Source: CAD feature listing. Evaluate the final solid. Frame: model axes, mm. A direction names the side the tool comes from. Coordinates: 2 decimals unless noted, no trailing zeros. Put each result on its own line as item: value.
from build123d import *

# Parameters (mm, degrees)
SKETCH2_R          = 3.937
CUT_EXTRUDE1_DEPTH = 89.486469768
CUT_EXTRUDE2_DEPTH = 89.486469768
SKETCH5_R          = 38.857978685
SKETCH5_R_2        = 10.795
CUT_EXTRUDE3_DEPTH = 1.27
SKETCH6_R          = 9.598574497
SKETCH6_R_2        = 5.136074626
CUT_EXTRUDE4_DEPTH = 0.508
FILLET3_R          = 2.54


with BuildPart() as part:
    # Sketch1 → Revolve1 (revolve)
    with BuildSketch(Plane(origin=(0, 0, 0), x_dir=(1, 0, 0), z_dir=(0, 1, 0))):
        with BuildLine():
            Line((0, 0), (-24.13, 0))
            Line((-24.13, 0), (-24.13, 48.133))
            ThreePointArc((-24.13, 48.133), (-12.065, 60.198), (0, 48.133))
            Line((0, 48.133), (0, 0))
        make_face()
    revolve(axis=Axis((0, 0, 0), (-1, 0, 0)))

    # Sketch2 → Cut-Extrude1 (cut, through all)
    with BuildSketch(Plane(origin=(0, 0, 0), x_dir=(0, 0, -1), z_dir=(1, 0, 0))):
        Circle(SKETCH2_R)
    extrude(amount=-CUT_EXTRUDE1_DEPTH, mode=Mode.SUBTRACT)

    # Sketch3 → Cut-Extrude2 (cut, through all)
    with BuildSketch(Plane(origin=(0, 0, 0), x_dir=(0, 0, -1), z_dir=(1, 0, 0))):
        with BuildLine():
            ThreePointArc((-7.868701987, 30.719014265), (-7.414350559, 33.395529437), (-5.121198299, 34.848671341))
            ThreePointArc((-5.121198299, 34.848671341), (0, 35.222955104), (5.121198299, 34.848671341))
            ThreePointArc((5.121198299, 34.848671341), (7.414350559, 33.395529437), (7.868701987, 30.719014265))
            Line((7.868701987, 30.719014265), (5.226080148, 20.402352367))
            ThreePointArc((5.226080148, 20.402352367), (3.322663277, 17.290224183), (0, 15.784154342))
            ThreePointArc((0, 15.784154342), (-3.322663277, 17.290224183), (-5.226080148, 20.402352367))
            Line((-5.226080148, 20.402352367), (-7.868701987, 30.719014265))
        make_face()
        with BuildLine():
            Line((-16.098624321, 29.076332472), (-9.794359632, 15.986465761))
            ThreePointArc((-9.794359632, 15.986465761), (-7.273828196, 15.104584389), (-6.391946824, 17.625115825))
            Line((-6.391946824, 17.625115825), (-12.696211514, 30.714982536))
            ThreePointArc((-12.696211514, 30.714982536), (-15.216742949, 31.596863908), (-16.098624321, 29.076332472))
        make_face()
        with BuildLine():
            ThreePointArc((-12.340172279, 9.840477432), (-15.589311763, 8.181733863), (-19.209232563, 8.633962814))
            Line((-19.209232563, 8.633962814), (-28.922771395, 13.000211347))
            ThreePointArc((-28.922771395, 13.000211347), (-30.732071739, 15.024217511), (-30.438426779, 17.7230953))
            ThreePointArc((-30.438426779, 17.7230953), (-27.538038696, 21.960371467), (-24.052396954, 25.730923416))
            ThreePointArc((-24.052396954, 25.730923416), (-21.486527816, 26.61776289), (-19.11066051, 25.304209225))
            Line((-19.11066051, 25.304209225), (-12.692417211, 16.805790793))
            ThreePointArc((-12.692417211, 16.805790793), (-11.446018427, 13.377259374), (-12.340172279, 9.840477432))
        make_face()
        with BuildLine():
            Line((-32.7697437, 5.541603622), (-18.605029061, 2.309077827))
            ThreePointArc((-18.605029061, 2.309077827), (-16.344020796, 3.729864614), (-17.764807583, 5.99087288))
            Line((-17.764807583, 5.99087288), (-31.929522221, 9.223398675))
            ThreePointArc((-31.929522221, 9.223398675), (-34.190530487, 7.802611888), (-32.7697437, 5.541603622))
        make_face()
        with BuildLine():
            ThreePointArc((-15.387190118, -3.513279694), (-16.116137508, -7.087768933), (-18.726688041, -9.635976839))
            Line((-18.726688041, -9.635976839), (-28.196651006, -14.508015872))
            ThreePointArc((-28.196651006, -14.508015872), (-30.907163058, -14.660636639), (-32.834146044, -12.748332988))
            ThreePointArc((-32.834146044, -12.748332988), (-34.33861956, -7.838819794), (-35.113293701, -2.762734656))
            ThreePointArc((-35.113293701, -2.762734656), (-34.20685948, -0.203722017), (-31.698552836, 0.834818527))
            Line((-31.698552836, 0.834818527), (-21.052512511, 0.554125976))
            ThreePointArc((-21.052512511, 0.554125976), (-17.594861779, -0.60905459), (-15.387190118, -3.513279694))
        make_face()
        with BuildLine():
            Line((-24.763824671, -22.166065784), (-13.404979114, -13.107092807))
            ThreePointArc((-13.404979114, -13.107092807), (-13.106079358, -10.45351929), (-15.759652875, -10.154619535))
            Line((-15.759652875, -10.154619535), (-27.118498432, -19.213592512))
            ThreePointArc((-27.118498432, -19.213592512), (-27.417398188, -21.867166029), (-24.763824671, -22.166065784))
        make_face()
        with BuildLine():
            ThreePointArc((-6.846586936, -14.221465552), (-4.506429979, -17.020037158), (-4.141812449, -20.649829394))
            Line((-4.141812449, -20.649829394), (-6.237124282, -31.091411229))
            ThreePointArc((-6.237124282, -31.091411229), (-7.807777183, -33.305732377), (-10.504330622, -33.620006517))
            ThreePointArc((-10.504330622, -33.620006517), (-15.280766495, -31.735219868), (-19.73241109, -29.175997183))
            ThreePointArc((-19.73241109, -29.175997183), (-21.167975243, -26.87180009), (-20.416035323, -24.263207549))
            Line((-20.416035323, -24.263207549), (-13.558883477, -16.114807003))
            ThreePointArc((-13.558883477, -16.114807003), (-10.493662321, -14.136738026), (-6.846586936, -14.221465552))
        make_face()
        with BuildLine():
            Line((1.890512446, -33.182235549), (1.890046539, -18.653355221))
            ThreePointArc((1.890046539, -18.653355221), (0.001760172, -16.765189956), (-1.886405093, -18.653476323))
            Line((-1.886405093, -18.653476323), (-1.885939187, -33.182356651))
            ThreePointArc((-1.885939187, -33.182356651), (0.00234718, -35.070521916), (1.890512446, -33.182235549))
        make_face()
        with BuildLine():
            ThreePointArc((6.850388874, -14.220597785), (10.497464259, -14.135870258), (13.562685415, -16.113939236))
            Line((13.562685415, -16.113939236), (20.419837261, -24.262339782))
            ThreePointArc((20.419837261, -24.262339782), (21.171777181, -26.870932322), (19.736213028, -29.175129416))
            ThreePointArc((19.736213028, -29.175129416), (15.284568432, -31.734352101), (10.50813256, -33.619138749))
            ThreePointArc((10.50813256, -33.619138749), (7.811579121, -33.30486461), (6.240926219, -31.090543462))
            Line((6.240926219, -31.090543462), (4.145614387, -20.648961626))
            ThreePointArc((4.145614387, -20.648961626), (4.510231917, -17.019169391), (6.850388874, -14.220597785))
        make_face()
        with BuildLine():
            Line((27.122008151, -19.211505151), (15.762581618, -10.153260695))
            ThreePointArc((15.762581618, -10.153260695), (13.109027277, -10.452330638), (13.408097219, -13.105884979))
            Line((13.408097219, -13.105884979), (24.767523753, -22.164129435))
            ThreePointArc((24.767523753, -22.164129435), (27.421078094, -21.865059493), (27.122008151, -19.211505151))
        make_face()
        with BuildLine():
            ThreePointArc((15.389635159, -3.511329838), (17.597306821, -0.607104734), (21.054957553, 0.556075831))
            Line((21.054957553, 0.556075831), (31.700997878, 0.836768383))
            ThreePointArc((31.700997878, 0.836768383), (34.209304522, -0.201772161), (35.115738743, -2.7607848))
            ThreePointArc((35.115738743, -2.7607848), (34.341064602, -7.836869939), (32.836591086, -12.746383132))
            ThreePointArc((32.836591086, -12.746383132), (30.9096081, -14.658686784), (28.199096048, -14.506066016))
            Line((28.199096048, -14.506066016), (18.729133083, -9.634026983))
            ThreePointArc((18.729133083, -9.634026983), (16.11858255, -7.085819077), (15.389635159, -3.511329838))
        make_face()
        with BuildLine():
            Line((31.930831552, 9.225880469), (17.766324261, 5.992446224))
            ThreePointArc((17.766324261, 5.992446224), (16.345682487, 3.73134684), (18.606781871, 2.310705066))
            Line((18.606781871, 2.310705066), (32.771289161, 5.544139311))
            ThreePointArc((32.771289161, 5.544139311), (34.191930935, 7.805238695), (31.930831552, 9.225880469))
        make_face()
        with BuildLine():
            ThreePointArc((12.340925299, 9.842041095), (11.446771448, 13.378823037), (12.693170232, 16.807354456))
            Line((12.693170232, 16.807354456), (19.111413531, 25.305772888))
            ThreePointArc((19.111413531, 25.305772888), (21.487280836, 26.619326553), (24.053149974, 25.732487079))
            ThreePointArc((24.053149974, 25.732487079), (27.538791716, 21.96193513), (30.4391798, 17.724658963))
            ThreePointArc((30.4391798, 17.724658963), (30.732824759, 15.025781174), (28.923524416, 13.00177501))
            Line((28.923524416, 13.00177501), (19.209985583, 8.635526477))
            ThreePointArc((19.209985583, 8.635526477), (15.590064784, 8.183297526), (12.340925299, 9.842041095))
        make_face()
        with BuildLine():
            Line((12.695840543, 30.715989922), (6.392415389, 17.625718912))
            ThreePointArc((6.392415389, 17.625718912), (7.274458414, 15.105244041), (9.794933285, 15.987287066))
            Line((9.794933285, 15.987287066), (16.098358439, 29.077558076))
            ThreePointArc((16.098358439, 29.077558076), (15.216315414, 31.598032947), (12.695840543, 30.715989922))
        make_face()
    extrude(amount=-CUT_EXTRUDE2_DEPTH, mode=Mode.SUBTRACT)

    # Sketch5 → Cut-Extrude3 (cut)
    with BuildSketch(Plane(origin=(0, 0, 0), x_dir=(0, 0, -1), z_dir=(1, 0, 0))):
        Circle(SKETCH5_R)
        Circle(SKETCH5_R_2, mode=Mode.SUBTRACT)
    cut_extrude3 = extrude(amount=-CUT_EXTRUDE3_DEPTH, mode=Mode.SUBTRACT)

    # Sketch6 → Cut-Extrude4 (cut)
    with BuildSketch(Plane.ZY.offset(24.13)):
        Circle(SKETCH6_R)
        Circle(SKETCH6_R_2, mode=Mode.SUBTRACT)
    cut_extrude4 = extrude(amount=-CUT_EXTRUDE4_DEPTH, mode=Mode.SUBTRACT)

    # Mirror8: Cut-Extrude3 across plane
    add(cut_extrude3.mirror(Plane(origin=(-12.065, 0, 0), x_dir=(0, 0, 1), z_dir=(1, 0, 0))), mode=Mode.SUBTRACT)

    # Mirror11: Cut-Extrude4 across plane
    add(cut_extrude4.mirror(Plane(origin=(-12.065, 0, 0), x_dir=(0, 0, 1), z_dir=(1, 0, 0))), mode=Mode.SUBTRACT)

    # Fillet3
    # the kernel refuses this fillet: 2.54 mm, written as the material it takes off along each edge
    with BuildSketch(Plane(origin=(0, 0, 0), x_dir=(0, 0, -1), z_dir=(0, -1, 0))) as fillet3_piece_1:
        with BuildLine():
            CenterArc((41.05768321, -2.54), FILLET3_R, 90, 60)
            Line((38.857978685, -1.27), (38.813984594, -1.2446))
            ThreePointArc((38.813984594, -1.2446), (38.807178685, -0.635), (38.807178685, 0))
            Line((38.807178685, 0), (38.857978685, 0.0508))
            Line((38.857978685, 0.0508), (41.05768321, 0.0508))
            Line((41.05768321, 0.0508), (41.05768321, 0))
        make_face()
    revolve(axis=Axis((0, 0, 0), (1, 0, 0)), mode=Mode.SUBTRACT)
    with BuildSketch(Plane(origin=(-24.13, 0, 0), x_dir=(0, 0, -1), z_dir=(0, -1, 0))) as fillet3_piece_2:
        with BuildLine():
            CenterArc((41.05768321, 2.54), FILLET3_R, 210, 60)
            Line((38.857978685, 1.27), (38.813984594, 1.2446))
            ThreePointArc((38.813984594, 1.2446), (38.807178685, 0.635), (38.807178685, 0))
            Line((38.807178685, 0), (38.857978685, -0.0508))
            Line((38.857978685, -0.0508), (41.05768321, -0.0508))
            Line((41.05768321, -0.0508), (41.05768321, 0))
        make_face()
    revolve(axis=Axis((-24.13, 0, 0), (1, 0, 0)), mode=Mode.SUBTRACT)


solid = part.part
1. Ray query, line 1 along Y through (x, z) = (-10.75, 3.5); line 2 along Y through (x, z) = (-9.5, 32.5); line 3 along Y through (x, z) = (-11.25, -23.5). Return the intervals inside material, ascending.
Numbers:
line 1: y = -60.02 to -1.8, 1.8 to 17.45, 35.05 to 60.02
line 2: y = -50.34 to -13.39, 0.76 to 5.48, 9.26 to 50.34
line 3: y = -55.39 to -21.15, -16.32 to -12.09, 0.62 to 3.43, 7.3 to 10.56, 26.15 to 55.39
2. First-contact query: pin 1 (11.5 mm diameter, centred on x = -8, y = -22.5, fed in from -Z); pin 2 (7.5 mm diameter, centred on x = -8.5, y = -24, fed in from +Z); pin 3 (5 mm diameter, centred on y = 10, z = 12.5, fed in from -X); pin 4 (9 mm diameter, centred on y = 0, z = 0, fed in from +X). Flat tips, straight axial feed; report the tip coordinate or a pass-through.
Numbers:
pin 1: stops at z = -57.55
pin 2: stops at z = 56.39
pin 3: stops at x = -22.86
pin 4: stops at x = 0
3. Cut plane A-A on x = -18.5. Count the separate pieces of the cut face and the enclosed holes in it, plus the area to 3 significant figures.
Numbers:
separate pieces: 1
enclosed holes: 15
area: 8,550 mm2
4. Set-up query: faces 1 (the flat face through (0, -22, -35)), 2 (the flat face through (-11.914, -12.104, -23.53)). Return all of +Z, -Z, +X, -X, +Y, -Y with unobstructed straight access to the full face (end or side cutting, diameter ignored); none if empty.
Numbers:
face 1: +Z, -Z, +X, +Y, -Y
face 2: +X, -X
5. Pull-direction query (Z, two-part tool) for faces 3 (the cylindrical face through (-11.914, -14.645, -30.946)), 4 (the flat face through (-23.622, -4, 4)), 5 (the flat face through (-24.13, 4, -1)); classes: pulls with the +Z half, pulls with the -Z half, needs draft (parallel to the pull), parting line crosses it, or undercut.
Numbers:
face 3: undercut
face 4: undercut
face 5: needs draft
